Input: part model. Units: mm. Frame: model coordinates. A direction names the side the tool comes from. Coordinates: 2 decimals unless noted, no trailing zeros. Write each loop counter-clockwise with the first axis right and the second up, starting at its lowest first coordinate (ties: lowest second). Pieces come first, ordered by that corner, then holes. Notation, with made-up numbers: (-27, 80.5) -> (-15, 80.5) arc R17 ccw to (-15, 89.5) -> close; hole circle Ø7 at (-11, 29). An arc over 180 degrees is marked (long way). One line per question, with ' | ' between items. Start each with the question number.
```python
from build123d import *

# Parameters (mm, degrees)
SCHIZZO1_R                   = 17
SCHIZZO1_R_2                 = 5.1
ESTRUSIONE_ESTRUSIONE1_DEPTH = 2
SCHIZZO2_R                   = 17
SCHIZZO2_R_2                 = 14.5
ESTRUSIONE_ESTRUSIONE2_DEPTH = 30
TAGLIO_ESTRUSIONE1_START     = -24
TAGLIO_ESTRUSIONE1_DEPTH     = 24
SCHIZZO4_W                   = 10
SCHIZZO4_H                   = 10
SCHIZZO4_R                   = 1.75
ESTRUSIONE_ESTRUSIONE4_DEPTH = 5
SCHIZZO6_W                   = 5
SCHIZZO6_H                   = 10
ESTRUSIONE_ESTRUSIONE5_DEPTH = 1
TAGLIO_ESTRUSIONE2_DEPTH     = 2.4
SCHIZZO8_R                   = 3.5
TAGLIO_ESTRUSIONE3_DEPTH     = 2.4
ESTRUSIONE_ESTRUSIONE6_DEPTH = 10
SCHIZZO10_R                  = 2.25
TAGLIO_ESTRUSIONE4_DEPTH     = 6
SCHIZZO11_R                  = 3.75
TAGLIO_ESTRUSIONE5_DEPTH     = 3


with BuildPart() as part:
    # Schizzo1 → Estrusione-Estrusione1 (new body)
    with BuildSketch(Plane.XY):
        Circle(SCHIZZO1_R)
        Circle(SCHIZZO1_R_2, mode=Mode.SUBTRACT)
    extrude(amount=ESTRUSIONE_ESTRUSIONE1_DEPTH)

    # Schizzo2 → Estrusione-Estrusione2 (add)
    with BuildSketch(Plane.XY.offset(2)):
        Circle(SCHIZZO2_R)
        Circle(SCHIZZO2_R_2, mode=Mode.SUBTRACT)
    extrude(amount=ESTRUSIONE_ESTRUSIONE2_DEPTH)

    # Schizzo3 → Taglio-Estrusione1 (cut)
    with BuildSketch(Plane.XY.offset(32).offset(TAGLIO_ESTRUSIONE1_START)):
        with BuildLine():
            Line((0, -17), (0, -14.5))
            ThreePointArc((0, -14.5), (-0.500297885, -14.491366465), (-1, -14.465476141))
            Line((-1, -14.465476141), (-1, -16.970562748))
            ThreePointArc((-1, -16.970562748), (-0.500216591, -16.992639094), (0, -17))
        make_face()
        with BuildLine():
            ThreePointArc((1, -14.465476141), (0.500297885, -14.491366465), (0, -14.5))
            Line((0, -14.5), (0, -17))
            ThreePointArc((0, -17), (0.500216591, -16.992639094), (1, -16.970562748))
            Line((1, -16.970562748), (1, -14.465476141))
        make_face()
    extrude(amount=TAGLIO_ESTRUSIONE1_DEPTH, mode=Mode.SUBTRACT)



with BuildPart() as body_2:
    # Schizzo4 → Estrusione-Estrusione4 (new body)
    with BuildSketch(Plane.ZY.offset(-1)):
        with Locations((20, -21.970562748)):
            Rectangle(SCHIZZO4_W, SCHIZZO4_H)
        with Locations(Location((20, -21.970562748, 0), (0, 0, 270))):
            Circle(SCHIZZO4_R, mode=Mode.SUBTRACT)
    estrusione_estrusione4 = extrude(amount=-ESTRUSIONE_ESTRUSIONE4_DEPTH)


with BuildPart() as part_1:
    add(part.part)

    add(body_2.part)  # Estrusione-Estrusione5 merges body 2
    # Schizzo6 → Estrusione-Estrusione5 (add)
    with BuildSketch(Plane(origin=(0, -16.970562748, 0), x_dir=(1, 0, 0), z_dir=(0, 1, 0))):
        with Locations((3.5, -20)):
            Rectangle(SCHIZZO6_W, SCHIZZO6_H)
    estrusione_estrusione5 = extrude(amount=ESTRUSIONE_ESTRUSIONE5_DEPTH)

    # Specchia4: Estrusione-Estrusione5 across plane
    add(estrusione_estrusione5.mirror(Plane(origin=(0, 0, 0), x_dir=(0, 0, 1), z_dir=(1, 0, 0))))

    # Specchia5: Estrusione-Estrusione4 across plane
    add(estrusione_estrusione4.mirror(Plane(origin=(0, 0, 0), x_dir=(0, 0, 1), z_dir=(1, 0, 0))))

    # Schizzo7 → Taglio-Estrusione2 (cut)
    with BuildSketch(Plane(origin=(6, 0, 0), x_dir=(0, 0, -1), z_dir=(1, 0, 0))):
        Polygon((-20, -18.679666214), (-22.85, -20.325114481), (-22.85, -23.616011016), (-20, -25.261459283), (-17.15, -23.616011016), (-17.15, -20.325114481), align=None)
    extrude(amount=-TAGLIO_ESTRUSIONE2_DEPTH, mode=Mode.SUBTRACT)

    # Schizzo8 → Taglio-Estrusione3 (cut)
    with BuildSketch(Plane.ZY.offset(6)):
        with Locations(Location((20, -21.970562748, 0), (0, 0, 270))):
            Circle(SCHIZZO8_R)
    extrude(amount=-TAGLIO_ESTRUSIONE3_DEPTH, mode=Mode.SUBTRACT)

    # Schizzo9 → Estrusione-Estrusione6 (add)
    with BuildSketch(Plane(origin=(0, 0, 0), x_dir=(-1, 0, 0), z_dir=(0, 0, -1))):
        with BuildLine():
            Line((-30, -60), (30, -60))
            Line((30, -60), (30, -54))
            Line((30, -54), (20, -54))
            Line((20, -54), (16.974272663, 0.934915801))
            ThreePointArc((16.974272663, 0.934915801), (0, -17), (-16.974272663, 0.934915801))
            Line((-16.974272663, 0.934915801), (-20, -54))
            Line((-20, -54), (-30, -54))
            Line((-30, -54), (-30, -60))
        make_face()
    extrude(amount=-ESTRUSIONE_ESTRUSIONE6_DEPTH)

    # Schizzo10 → Taglio-Estrusione4 (cut)
    with BuildSketch(Plane(origin=(0, -54, 0), x_dir=(1, 0, 0), z_dir=(0, 1, 0))):
        with Locations(Location((25, -5, 0), (0, 0, 270))):
            Circle(SCHIZZO10_R)
        with Locations(Location((-25, -5, 0), (0, 0, 270))):
            Circle(SCHIZZO10_R)
    extrude(amount=-TAGLIO_ESTRUSIONE4_DEPTH, mode=Mode.SUBTRACT)

    # Schizzo11 → Taglio-Estrusione5 (cut)
    with BuildSketch(Plane(origin=(0, -54, 0), x_dir=(1, 0, 0), z_dir=(0, 1, 0))):
        with Locations(Location((-25, -5, 0), (0, 0, 270))):
            Circle(SCHIZZO11_R)
        with Locations(Location((25, -5, 0), (0, 0, 270))):
            Circle(SCHIZZO11_R)
    extrude(amount=-TAGLIO_ESTRUSIONE5_DEPTH, mode=Mode.SUBTRACT)


solid = part_1.part
```
1) Section A-A, the plane x = 0. Return loops of the section in (y, z), then the cut area to 3 significant figures.
2) First-contact query: P1, Ø2, axis at x = -8.5, y = -34.5, coming from the +Z side; P2, Ø5.5, axis at x = -4.5, y = -23.5, coming from the +Z side; P3, Ø5, axis at y = -22, z = 17.5, coming from the -X side. Flat tips, straight axial feed; report the tip coordinate or a pass-through.
3) Pull-direction query (X, two-part tool) for faces 1 (the face through (-1, -19, 20)), 2 (the face through (6, -19, 19)), 3 (the face through (4.817, -24.45, 18.595)); classes: released by +X, released by -X, zero draft, split by the parting line, or undercut.
4) Ray query, line 1 (X direction, y = -55.8, z = 5); line 2 (X direction, y = 0, z = 12.25); line 3 (X direction, y = -10.5, z = 3.5). Return the intervals inside material, ascending.
5) Section B-B, the plane z = 4. Return loops of the section in (x, y).
6) Access query for faces 4 (the face through (5, -22, 17.15)), 5 (the face through (-28.4, -54, 2.7)), 6 (the face through (-27, -57, 7)), 7 (the face through (0, -16, 8)), 8 (the face through (-3, -26.971, 20)). Directions: +Z, -Z, +X, -X, +Y, -Y. A direction counts if a zero-diameter tool reaches every point of the face in a straight line with its end or side. Return the directions, or none.
7) Section D-D, the plane x = -25. Return loops of the section in (y, z).
Answer block:
1) outline: (-60, 0) -> (-5.1, 0) -> (-5.1, 2) -> (-14.5, 2) -> (-14.5, 8) -> (-17, 8) -> (-17, 10) -> (-60, 10) -> close; (5.1, 0) -> (17, 0) -> (17, 32) -> (14.5, 32) -> (14.5, 2) -> (5.1, 2) -> close | area: 568 mm2
2) P1: stops at z = 10 | P2: stops at z = 25 | P3: stops at x = -6
3) face 1: undercut | face 2: released by +X | face 3: zero draft
4) line 1: x = -30 to -28.75, -21.25 to 21.25, 28.75 to 30 | line 2: x = -17 to -14.5, 14.5 to 17 | line 3: x = -17.6 to -10, 10 to 17.6
5) outline: (-30, -60) -> (-27.02, -60) -> (-27.02, -57) -> (-28.61, -57) -> (-28.61, -54) -> (-30, -54) -> close; (-22.98, -60) -> (22.98, -60) -> (22.98, -57) -> (21.39, -57) -> (21.39, -54) -> (20, -54) -> (16.97, 0.93) arc R17 ccw to (-16.97, 0.93) -> (-20, -54) -> (-21.39, -54) -> (-21.39, -57) -> (-22.98, -57) -> close; (27.02, -60) -> (30, -60) -> (30, -54) -> (28.61, -54) -> (28.61, -57) -> (27.02, -57) -> close; hole circle Ø29 at (0, 0)
6) face 4: +X | face 5: +Z, -Z, -X, +Y | face 6: +Y | face 7: +Z | face 8: +Z, +X, -X, -Y
7) outline: (-60, 0) -> (-54, 0) -> (-54, 1.25) -> (-57, 1.25) -> (-57, 2.75) -> (-60, 2.75) -> close; (-60, 7.25) -> (-57, 7.25) -> (-57, 8.75) -> (-54, 8.75) -> (-54, 10) -> (-60, 10) -> close
